Geometry: final body of the model. Coordinates: model frame, mm. A direction names the side the tool comes from. Give positions to 0.01 mm unless a question says otherwise; leave off trailing zeros. Write each loop counter-clockwise with the first axis right and the second up, starting at its lowest first coordinate (ties: lowest second). Pieces come first, ordered by that corner, then holes. Notation, with made-up numbers: M 29,32 L 85,32 A22 ccw 85,50 Z; hole C 77.5,81.25 d5. An arc over 180 degrees is marked long. Use a Markdown table: item, result. Add a question column.
(1) Cut plane C-C (x = 95). Output: boundary loops of the cut face in (y, z), plus the area to 3 significant figures.
(2) Reachability of faces 1 (the flat face through (91, 1, 25)), 2 (the flat face through (-93.312, -4, 25)), 3 (the flat face through (-94.812, -4, 25)) from +Z, -Z, +X, -X, +Y, -Y: full face, straight path, thin tool, end or side. Return the list, or none.
(3) Draft query along Y for faces 4 (the flat face through (0, -55, 1)), 5 (the cylindrical face through (96.847, -48.766, 0.74)), 6 (the flat face through (83, -1, 13)). Return one class per face: released by +Y, released by -Y, zero draft, split by the parting line, or undercut.
(4) Pin query (flat end, axial travel): pin 1 Ø1 at (x, z) = (13, 37) entering from -Y; pin 2 Ø13 at (x, z) = (93.5, 18) entering from -Y; pin 3 Ø1.5 at (x, y) = (-77, 23.5) entering from +Z. Return the tip coordinate at first contact, or that it passes through.
(5) Cut plane D-D (z = 30). Output: boundary loops of the cut face in (x, y).
(6) Cut plane B-B (y = 20.5). Output: boundary loops of the cut face in (x, z).
(7) Cut plane A-A (z = 14). Output: boundary loops of the cut face in (x, y).
(8) Material intervals for L1, parallel to Z at x = -93.8, y = -50; L2, parallel to X at y = -15.5, z = 17; L3, parallel to Y at x = 95, z = 0.7, sorted ascending.
```python
from build123d import *

# Parameters (mm, degrees)
F0_R     = 2
F0_W     = 16
F0_H     = 88
F2_DEPTH = 1.5
F0_W_2   = 1.5
F0_H_2   = 104
F3_DEPTH = 50
F4_DEPTH = 25
F5_D     = 4


# Not quite as in the source:
# - the program builds the solid bodies; features that only make, move or delete a surface that nothing else refers to are left out


with BuildPart() as f2:
    # F0 (on Top) → F2 (new body)
    with BuildSketch(Plane.XY):
        Polygon((100, 53.5), (-100, 53.5), (-100, -55), (-94.811744988, -55), (-94.811744988, 49), (-93.311744988, 49), (-93.311744988, -55), (100, -55), align=None)
        with Locations((95, -48)):
            Circle(F0_R, mode=Mode.SUBTRACT)
        with Locations((91, 0)):
            Rectangle(F0_W, F0_H, mode=Mode.SUBTRACT)
        with Locations((91, 0)):
            Rectangle(F0_W, F0_H)
    extrude(amount=F2_DEPTH)

    # F0 (on Top) → F3 (join)
    with BuildSketch(Plane.XY):
        Polygon((-58.6367584765, 55), (-100, 55), (-100, 53.5), (100, 53.5), (100, 55), (72.2615793347, 55), align=None)
        with Locations((-94.061744988, -3)):
            Rectangle(F0_W_2, F0_H_2)
    extrude(amount=F3_DEPTH)

    # F0 (on Top) → F4 (join)
    with BuildSketch(Plane.XY):
        with Locations((91, 0)):
            Rectangle(F0_W, F0_H)
    extrude(amount=F4_DEPTH)

    # F5 (through all)
    with Locations(Plane.YZ):
        with Locations((-50, 30)):
            Hole(F5_D / 2)


solid = f2.part
```
Answer list:
| question | item | result |
|---|---|---|
| 1 | outline | M -55,0 L -50,0 L -50,1.5 L -55,1.5 Z; M -46,0 L 55,0 L 55,50 L 53.5,50 L 53.5,1.5 L 44,1.5 L 44,25 L -44,25 L -44,1.5 L -46,1.5 Z |
| 1 | area | 2,300 mm² |
| 2 | face 1 | +Z, +X, -Y |
| 2 | face 2 | +Z, -Y |
| 2 | face 3 | +Z, -X, -Y |
| 3 | face 4 | released by -Y |
| 3 | face 5 | undercut |
| 3 | face 6 | zero draft |
| 4 | pin 1 | y = 53.5 |
| 4 | pin 2 | y = -44 |
| 4 | pin 3 | z = 1.5 |
| 5 | outline | M -100,53.5 L 100,53.5 L 100,55 L -100,55 Z; M -94.81,-55 L -93.31,-55 L -93.31,-52 L -94.81,-52 Z; M -94.81,-48 L -93.31,-48 L -93.31,49 L -94.81,49 Z |
| 6 | outline | M -100,0 L 100,0 L 100,1.5 L 99,1.5 L 99,25 L 83,25 L 83,1.5 L -93.31,1.5 L -93.31,50 L -94.81,50 L -94.81,1.5 L -100,1.5 Z |
| 7 | outline | M -100,53.5 L 100,53.5 L 100,55 L -100,55 Z; M -94.81,-55 L -93.31,-55 L -93.31,49 L -94.81,49 Z; M 83,-44 L 99,-44 L 99,44 L 83,44 Z |
| 8 | L1 | 0 to 28, 32 to 50 |
| 8 | L2 | -94.81 to -93.31, 83 to 99 |
| 8 | L3 | -55 to -50, -46 to 55 |
